Could you check a few things on this drawing? It's one solid part, dimensions in mm from its lowest x, y, z. A direction names the side the tool comes from. Coordinates: 2 decimals unless noted, no trailing zeros. Write each loop counter-clockwise with the first axis right and the second up, starting at its lowest first coordinate (ties: lowest second). Pieces come first, ordered by that corner, then holes.
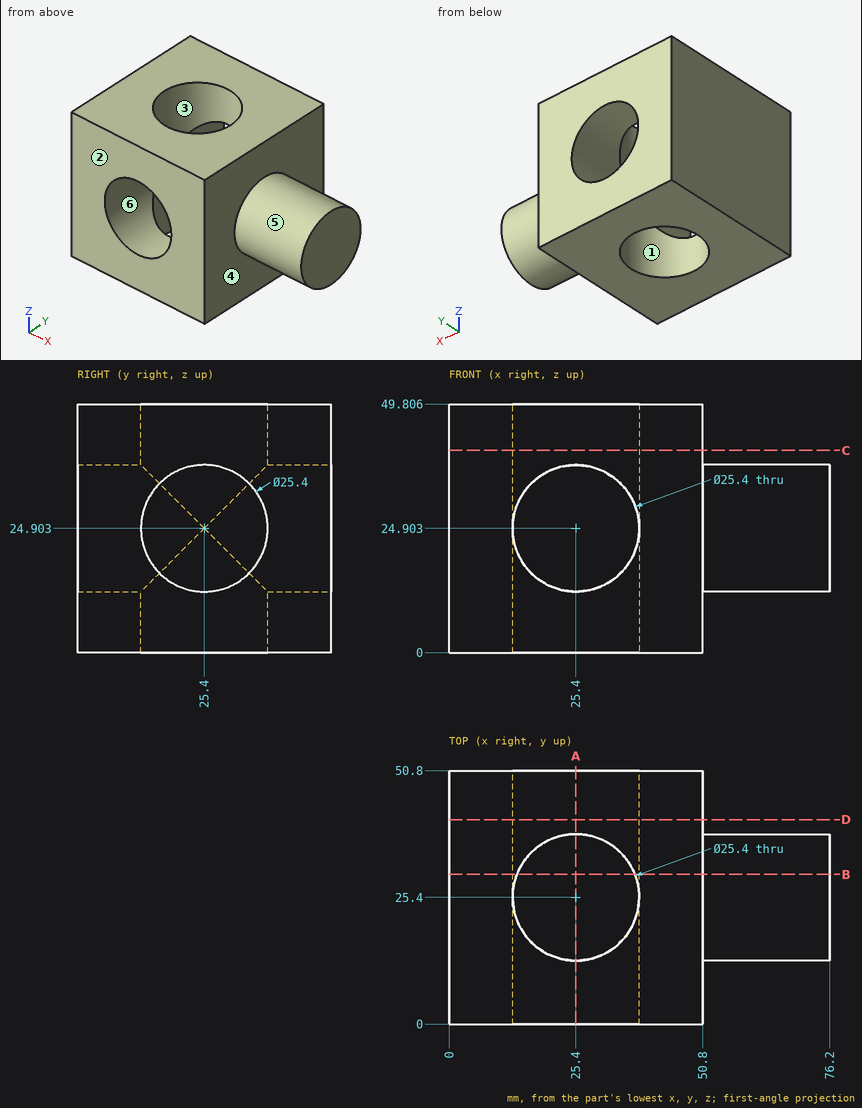
1) We'd pull the mould along Y, two halves only. Please class the marked faces 1, 2, 3 and 4: pulls with the +Y half, pulls with the -Y half, needs draft (parallel to the pull), parting line crosses it, or undercut.
Values follow:
face 1: undercut
face 2: pulls with the -Y half
face 3: undercut
face 4: needs draft
2) Imagine slicing it at B-B on y = 30. Please give me the cut outline in (x, z) (1 decimal), then the cut area to 3 significant figures.
Values follow:
outline: (0, 0) - (13.6, 0) - (13.6, 20.3) arc R12.7 cw to (13.6, 29.5) - (13.6, 49.8) - (0, 49.8) - close; (37.2, 0) - (50.8, 0) - (50.8, 13.1) - (76.2, 13.1) - (76.2, 36.7) - (50.8, 36.7) - (50.8, 49.8) - (37.2, 49.8) - (37.2, 29.5) arc R12.7 cw to (37.2, 20.3) - close
area: 1,940 mm2
3) Will these pins go through, and if not, where does the flat tip stop? pin 1 (5 mm diameter, centred on x = 58.5, z = 21, fed in from +Y); pin 2 (3 mm diameter, centred on x = 66.5, y = 25.5, fed in from +Z).
Values follow:
pin 1: stops at y = 38.02
pin 2: stops at z = 37.6
4) Imagine slicing it at C-C on z = 40.5. Please give me the cut outline in (x, y).
Values follow:
outline: (0, 0) - (50.8, 0) - (50.8, 50.8) - (0, 50.8) - close; hole circle Ø25.4 at (25.4, 25.4)
5) Imagine slicing it at A-A on x = 25.4. Please give me the cut outline in (y, z), then the cut area to 3 significant figures.
Values follow:
outline: (0, 0) - (12.7, 0) - (12.7, 12.2) - (0, 12.2) - close; (0, 37.6) - (12.7, 37.6) - (12.7, 49.81) - (0, 49.81) - close; (38.1, 0) - (50.8, 0) - (50.8, 12.2) - (38.1, 12.2) - close; (38.1, 37.6) - (50.8, 37.6) - (50.8, 49.81) - (38.1, 49.81) - close
area: 620 mm2
6) On a 3-axis mill with a long thin cutter (end or side, diameter ignored), from which of +Z, -Z, +X, -X, +Y, -Y can I reach the whole of each face in a straight line? I mean the marked faces 5 and 6. Say none if no direction works.
Values follow:
face 5: +X
face 6: +Y, -Y
7) I need wall thicknesses on probe 1 along X at (y, z) = (25, 13); probe 2 along Y at (x, z) = (25, 41); probe 3 along Z at (x, y) = (25.4, 11.75). Which ranges of each line are inside material? Lowest first, please.
Values follow:
probe 1: x = 0 to 12.71, 38.09 to 76.2
probe 2: y = 0 to 12.71, 38.09 to 50.8
probe 3: z = 0 to 12.2, 37.6 to 49.81
8) Imagine slicing it at D-D on y = 41. Please give me the cut outline in (x, z).
Values follow:
outline: (0, 0) - (50.8, 0) - (50.8, 49.81) - (0, 49.81) - close; hole circle Ø25.4 at (25.4, 24.9)
